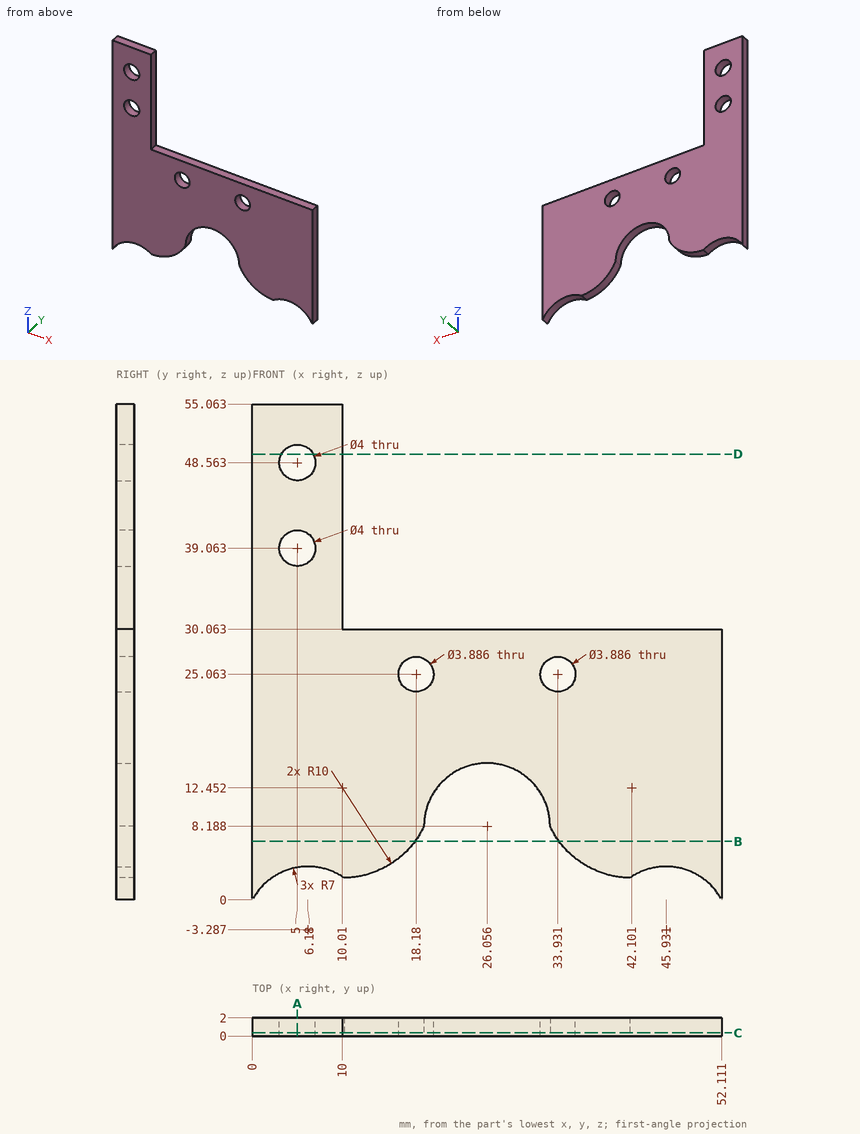
Input: dimensioned drawing with shaded views. Units: mm. Origin: part minimum x, y, z. Coordinates: 2 decimals unless noted, no trailing zeros. Loops run counter-clockwise (first coordinate to the right, second up) from the corner with the lowest first, then second, coordinate; pieces in that order, holes last. Notation, with made-up numbers: (-9.5, 42.5) -> (18.5, 42.5) arc R9 ccw to (18.5, 55.5) -> close; hole circle Ø2 at (-7, 44). An arc over 180 degrees is marked (long way). Use a Markdown table: item, result. Add a question column.
(1) Section query C-C, the plane y = 0.35. Return loops of the section in (x, z) (1 decimal).
(2) Pin query (flat end, axial travel): pin 1 Ø2.5 at (x, z) = (5, 39.06) entering from +Y; pin 2 Ø1 at (y, z) = (1.5, 43) entering from +X. Return the tip coordinate at first contact, or that it passes through.
(3) Section query A-A, the plane x = 5. Return loops of the section in (y, z).
(4) Section query D-D, the plane z = 49.5. Return loops of the section in (x, y).
(5) Section query B-B, the plane z = 6.5. Return loops of the section in (x, y) (1 decimal).
(6) Line query: line 1 along Z through (x, y) = (4.5, 1.6); line 2 along X through (y, z) = (1.45, 26) (1 decimal); line 3 along Z through (x, y) = (26, 0.6). Output: solid intervals per line, ascending.
Answer:
| question | item | result |
|---|---|---|
| 1 | outline | (0, 0) arc R7 cw to (10.2, 2.5) arc R10 ccw to (19.1, 8.2) arc R7 cw to (33.1, 8.2) arc R10 ccw to (41.9, 2.5) arc R7 cw to (52.1, 0) -> (52.1, 30.1) -> (10, 30.1) -> (10, 55.1) -> (0, 55.1) -> close; hole circle Ø4 at (5, 39.1); hole circle Ø4 at (5, 48.6); hole circle Ø3.9 at (18.2, 25.1); hole circle Ø3.9 at (33.9, 25.1) |
| 2 | pin 1 | passes through |
| 2 | pin 2 | stops at x = 10 |
| 3 | outline | (0, 3.61) -> (2, 3.61) -> (2, 37.06) -> (0, 37.06) -> close; (0, 41.06) -> (2, 41.06) -> (2, 46.56) -> (0, 46.56) -> close; (0, 50.56) -> (2, 50.56) -> (2, 55.06) -> (0, 55.06) -> close |
| 4 | outline | (0, 0) -> (3.23, 0) -> (3.23, 2) -> (0, 2) -> close; (6.77, 0) -> (10, 0) -> (10, 2) -> (6.77, 2) -> close |
| 5 | outline | (0, 0) -> (18, 0) -> (18, 2) -> (0, 2) -> close; (34.1, 0) -> (52.1, 0) -> (52.1, 2) -> (34.1, 2) -> close |
| 6 | line 1 | z = 3.51 to 37.13, 41 to 46.63, 50.5 to 55.06 |
| 6 | line 2 | x = 0 to 16.5, 19.9 to 32.2, 35.6 to 52.1 |
| 6 | line 3 | z = 15.19 to 30.06 |
